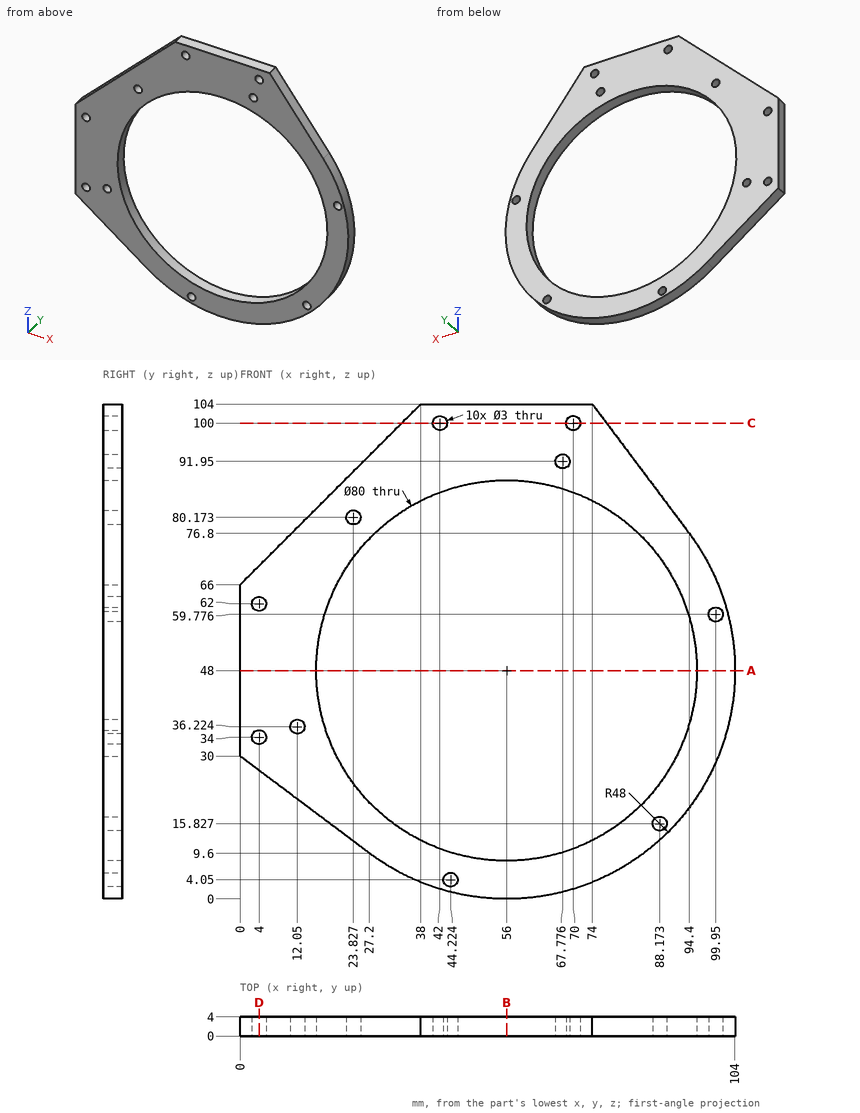
Print and shaded views of the part. All mm, measured from the part's lowest x, y and z. Give positions to 0.01 mm unless a question says otherwise; leave off trailing zeros. Write each loop counter-clockwise with the first axis right and the second up, starting at its lowest first coordinate (ties: lowest second). Pieces come first, ordered by that corner, then holes. Notation, with made-up numbers: (-20, 61.25) -> (3, 61.25) arc R9 ccw to (3, 71.25) -> close; hole circle Ø7 at (3, 0). An arc over 180 degrees is marked (long way). Write item = value, one per line.
(1) Slice it at C-C, the plane z = 100. Give the cut face in (x, y), then the cut area to 3 significant figures.
Determined:
outline = (34, 0) -> (40.5, 0) -> (40.5, 4) -> (34, 4) -> close; (43.5, 0) -> (68.5, 0) -> (68.5, 4) -> (43.5, 4) -> close; (71.5, 0) -> (77, 0) -> (77, 4) -> (71.5, 4) -> close
area = 148 mm2
(2) Probe line 1 along Z through (x, y) = (89.5, 1.85) (1 decimal); line 2 along X through (y, z) = (1.9, 60) (1 decimal); line 3 along Z through (x, y) = (70, 3.2). List the from-to ranges inside material, lowest first.
Determined:
line_1 = 13.6 to 15.1, 16.5 to 26.1, 69.9 to 83.3
line_2 = 0 to 17.8, 94.2 to 98.5, 101.4 to 102.5
line_3 = 2.09 to 10.53, 85.47 to 98.5, 101.5 to 104
(3) Flat gauge pins, fed straight in: P1, Ø1.8, axis at x = 70, z = 100, coming from the -Y side; P2, Ø2, axis at y = 2.5, z = 90.5, coming from the +X side (1 decimal). Where does each tip first touch, or does it go through?
Determined:
P1 = through
P2 = 84.9
(4) Slice it at A-A, the plane z = 48. Give the cut face in (x, y), then the cut area to 3 significant figures.
Determined:
outline = (0, 0) -> (16, 0) -> (16, 4) -> (0, 4) -> close; (96, 0) -> (104, 0) -> (104, 4) -> (96, 4) -> close
area = 96.0 mm2
(5) Slice it at D-D, the plane x = 4. Give the cut face in (y, z).
Determined:
outline = (0, 27) -> (4, 27) -> (4, 32.5) -> (0, 32.5) -> close; (0, 35.5) -> (4, 35.5) -> (4, 60.5) -> (0, 60.5) -> close; (0, 63.5) -> (4, 63.5) -> (4, 70) -> (0, 70) -> close
(6) Slice it at B-B, the plane x = 56. Give the cut face in (y, z), then the cut area to 3 significant figures.
Determined:
outline = (0, 0) -> (4, 0) -> (4, 8) -> (0, 8) -> close; (0, 88) -> (4, 88) -> (4, 104) -> (0, 104) -> close
area = 96.0 mm2
